Input: part model. Units: mm. Frame: model coordinates. A direction names the side the tool comes from. Coordinates: 2 decimals unless noted, no trailing zeros. Loops run counter-clockwise (first coordinate to the right, second up) from the corner with the lowest first, then second, coordinate; pieces in that order, holes last.
Item 1: Reachability of faces 3 (the cylindrical face through (3.698, -6.441, -3.037)), 4 (the cylindrical face through (3.698, 1.886, 6.894)), 5 (the cylindrical face through (3.7, 5.83, 2.11)) from +Z, -Z, +X, -X, +Y, -Y: full face, straight path, thin tool, end or side. Return the list, or none.
Item 2: Ray query, line 1 along Y through (x, z) = (4.75, 7); line 2 along Z through (x, y) = (1.5, -5) (3 decimals); line 3 along Z through (x, y) = (2, 2.75). Return the intervals inside material, ascending.
Item 3: Section B-B on y = 1. Return loops of the section in (x, z), and give its area (3 significant figures).
Item 4: Pull-direction query (Z, two-part tool) for faces 1 (the cylindrical face through (3.7, 5.82, -2.13)), 2 (the cylindrical face through (3.7, -1.87, 6.87)); classes: released by +Z, released by -Z, zero draft, split by the parting line, or undercut.
Item 5: Contact query for flat-ended pins moving along their axis: P1, Ø2, axis at x = 3.5, y = 6, coming from the -Z side (3 decimals); P2, Ø2, axis at x = 3, y = 3.5, coming from the +Z side; P3, Ø1.5, axis at x = 4, y = -1.5, coming from the +Z side. Output: stop coordinate, or through.
Item 6: Section C-C on y = -3.25. Return loops of the section in (x, z).
Item 7: Section A-A on z = 2.25. Return loops of the section in (x, y), and give its area (3 significant figures).
```python
from build123d import *

# Parameters (mm, degrees)
BASPROSKE_W              = 7.5
BASPROSKE_H              = 8
TOOTHCUT_DEPTH           = 14.57387196
TEETHCUTS_COUNT          = 18
TEETHCUTS_ANGLE          = 340
BORSKE_R                 = 2.5
BORE_DEPTH               = 50.0000508
TAGLIO_ESTRUSIONE1_DEPTH = 10


with BuildPart() as part:
    # BasProSke → Base-Revolve (revolve)
    with BuildSketch(Plane(origin=(0, 0, 0), x_dir=(1, 0, 0), z_dir=(0, 1, 0)), mode=Mode.PRIVATE) as base_revolve_sk:
        with Locations((3.75, 4)):
            Rectangle(BASPROSKE_W, BASPROSKE_H)
    revolve(base_revolve_sk.sketch.rotate(Axis((-10, 0, 0), (1, 0, 0)), 180), axis=Axis((-10, 0, 0), (1, 0, 0)))

    # TooCutSke → ToothCut (cut, through all)
    with BuildSketch(Plane(origin=(0, 0, 0), x_dir=(0, 0, -1), z_dir=(1, 0, 0))):
        with BuildLine():
            ThreePointArc((0.478981505, 6.180467435), (0, 6.199), (-0.478981505, 6.180467435))
            ThreePointArc((-0.478981505, 6.180467435), (-0.660732846, 7.117783932), (-1.138936203, 7.944172045))
            ThreePointArc((-1.138936203, 7.944172045), (0, 8.0254), (1.138936203, 7.944172045))
            ThreePointArc((1.138936203, 7.944172045), (0.660732846, 7.117783932), (0.478981505, 6.180467435))
        make_face()
    toothcut = extrude(amount=TOOTHCUT_DEPTH, mode=Mode.SUBTRACT)

    # TeethCuts: ToothCut ×18 about axis
    teethcuts_axis = Axis((-10, 0, 0), (1, 0, 0))
    for i in range(1, TEETHCUTS_COUNT):
        add(toothcut.rotate(teethcuts_axis, i * TEETHCUTS_ANGLE / (TEETHCUTS_COUNT - 1)), mode=Mode.SUBTRACT)

    # BorSke → Bore (cut, symmetric)
    with BuildSketch(Plane(origin=(0, 0, 0), x_dir=(0, 0, -1), z_dir=(1, 0, 0))):
        with Locations(Location((0, 0, 0), (0, 0, 180))):
            Circle(BORSKE_R)
    extrude(amount=BORE_DEPTH, both=True, mode=Mode.SUBTRACT)

    # Schizzo2 → Taglio-Estrusione1 (cut)
    with BuildSketch(Plane(origin=(7.5, 0, 0), x_dir=(0, 0, -1), z_dir=(1, 0, 0))):
        Polygon((0, 2.886751346), (-2.5, 1.443375673), (-2.5, -1.443375673), (0, -2.886751346), (2.5, -1.443375673), (2.5, 1.443375673), align=None)
    extrude(amount=-TAGLIO_ESTRUSIONE1_DEPTH, mode=Mode.SUBTRACT)


solid = part.part
```
Results found:
1. face 3: +X, -X, -Y
1. face 4: +Z, +X, -X
1. face 5: +X, -X
2. line 1: y = -3.03 to -1.95, -0.61 to 0.61, 1.95 to 3.03
2. line 2: z = -6.245 to -5.033, -3.664 to 3.664, 5.033 to 6.245
2. line 3: z = -7.51 to -5.74, -5.56 to -0.24, 0.24 to 5.56, 5.74 to 7.51
3. outline: (0, -6.12) - (7.5, -6.12) - (7.5, -2.5) - (0, -2.5) - close; (0, 2.5) - (7.5, 2.5) - (7.5, 6.12) - (0, 6.12) - close
3. area: 54.3 mm2
4. face 1: undercut
4. face 2: released by +Z
5. P1: stops at z = -6.245
5. P2: stops at z = 7.6
5. P3: stops at z = 7.38
6. outline: (0, -5.28) - (7.5, -5.28) - (7.5, 5.28) - (0, 5.28) - close
7. outline: (0, -5.78) - (7.5, -5.78) - (7.5, -1.59) - (0, -1.59) - close; (0, 1.59) - (7.5, 1.59) - (7.5, 5.78) - (0, 5.78) - close
7. area: 62.8 mm2
